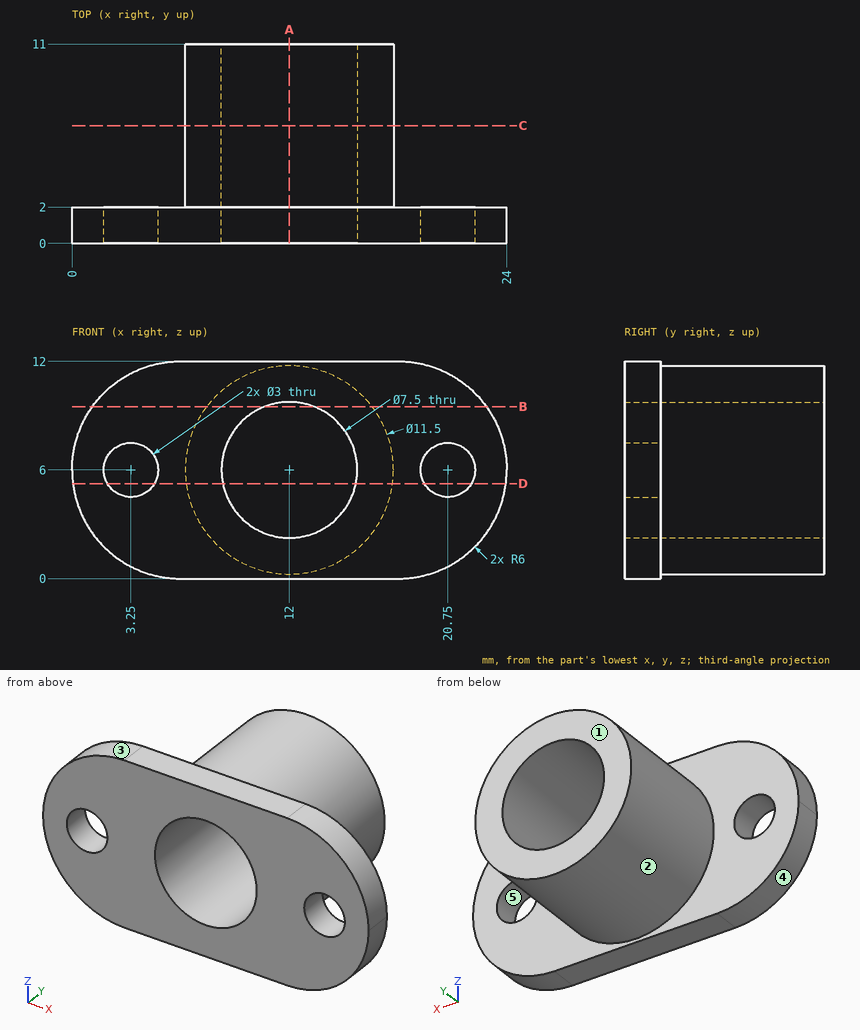
Here's the drawing with two shaded views (mm, measured from the low corner). I have some questions. A direction names the side the tool comes from. Round coordinates to 2 decimals unless told otherwise and drop trailing zeros. Write each loop counter-clockwise with the first axis right and the second up, starting at its lowest first coordinate (ties: lowest second). Pieces come first, ordered by that corner, then holes.
(1) Suppose I cut it at B-B on z = 9.5. Write out the boundary of the cut face in (x, y), and give its area (3 significant figures).
Findings below:
outline: (1.13, 0) - (10.65, 0) - (10.65, 11) - (7.44, 11) - (7.44, 2) - (1.13, 2) - close; (13.35, 0) - (22.87, 0) - (22.87, 2) - (16.56, 2) - (16.56, 11) - (13.35, 11) - close
area: 96.0 mm2
(2) Suppose I cut it at C-C on y = 6.5. Write out the boundary of the cut face in (x, z), and give its area (3 significant figures).
Findings below:
outline: circle Ø11.5 at (12, 6); hole circle Ø7.5 at (12, 6)
area: 59.7 mm2
(3) For pin 1 (6 mm diameter, centred on x = 12, z = 6, fed in from +Y); pin 2 (1 mm diameter, centred on y = 1.5, z = 10.5, fed in from -X); pin 3 (5 mm diameter, centred on y = 7, z = 9, fed in from +X); pin 4 (6 mm diameter, centred on x = 14, y = 6.5, fed in from +Z), each with a flat end and sliding along its axis, tell me the tip position at first contact or that it passes through.
Findings below:
pin 1: passes through
pin 2: stops at x = 1.53
pin 3: stops at x = 17.73
pin 4: stops at z = 11.75
(4) Thinking about a two-plate mould opening in Z: for the marked faces 3, 4 and 5, which applies, +Z half, -Z half, draft (parallel to the pull), parting line (faces both ways), or undercut?
Findings below:
face 3: +Z half
face 4: -Z half
face 5: undercut
(5) If I drill on probe 1 along Z at (x, y) = (12, 7); probe 2 along Z at (x, y) = (9.75, 10); probe 3 along Y at (x, z) = (17.25, 3), over which ranges is the centre line in solid material (lowest first)?
Findings below:
probe 1: z = 0.25 to 2.25, 9.75 to 11.75
probe 2: z = 0.71 to 3, 9 to 11.29
probe 3: y = 0 to 2
(6) Suppose I cut it at D-D on z = 5.25. Write out the boundary of the cut face in (x, y), and give its area (3 significant figures).
Findings below:
outline: (0.05, 0) - (1.95, 0) - (1.95, 2) - (0.05, 2) - close; (4.55, 0) - (8.33, 0) - (8.33, 11) - (6.3, 11) - (6.3, 2) - (4.55, 2) - close; (15.67, 0) - (19.45, 0) - (19.45, 2) - (17.7, 2) - (17.7, 11) - (15.67, 11) - close; (22.05, 0) - (23.95, 0) - (23.95, 2) - (22.05, 2) - close
area: 59.2 mm2
(7) Which directions (+Z, -Z, +X, -X, +Y, -Y) give clear straight access to the entire face, cutting with the end or side of a thin tool? Please do the marked faces 1 and 2.
Findings below:
face 1: +Z, -Z, +X, -X, +Y
face 2: +Y
(8) Suppose I cut it at A-A on x = 12. Write out the boundary of the cut face in (y, z).
Findings below:
outline: (0, 0) - (2, 0) - (2, 0.25) - (11, 0.25) - (11, 2.25) - (0, 2.25) - close; (0, 9.75) - (11, 9.75) - (11, 11.75) - (2, 11.75) - (2, 12) - (0, 12) - close
